```python
from build123d import *

# Parameters (mm, degrees)
F1_DEPTH = 25
F3_DEPTH = 30
F4_W     = 5
F4_H     = 10
F5_DEPTH = 15.001


with BuildPart() as f1:
    # F0 (on Front) → F1 (new body)
    with BuildSketch(Plane.XZ):
        Polygon((0, 80), (0, 0), (15, 0), (15, 35), (75, 35), (75, 80), align=None)
    extrude(amount=-F1_DEPTH)

    # F2 (on face) → F3 (cut)
    with BuildSketch(Plane.XY.offset(80)):
        with BuildLine():
            ThreePointArc((50, 0), (25, 5.456439), (0, 0))
            Line((0, 0), (50, 0))
        make_face()
    extrude(amount=-F3_DEPTH, mode=Mode.SUBTRACT)

    # F4 (on face) → F5 (cut, through all)
    with BuildSketch(Plane.YZ.offset(15)):
        with Locations((22.5, 5)):
            Rectangle(F4_W, F4_H)
    extrude(amount=-F5_DEPTH, mode=Mode.SUBTRACT)


solid = f1.part
```
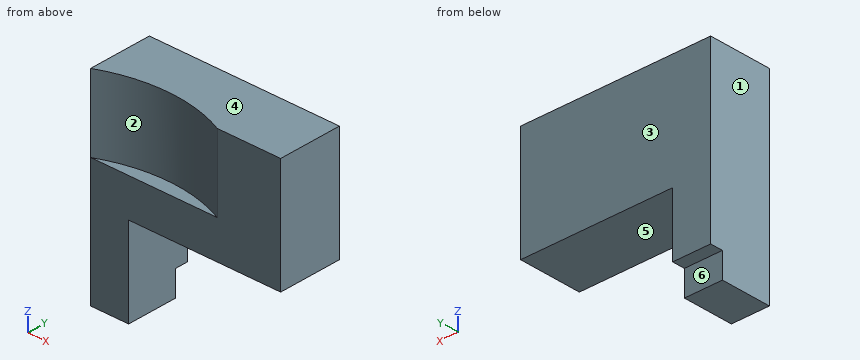
Source: CAD feature listing. Evaluate the final solid. Frame: model axes, mm. Face numbers are marked on the shaded views. A direction names the side the tool comes from. Give positions to 0.01 mm unless a question says otherwise; leave off trailing zeros. Write each loop counter-clockwise with the first axis right and the second up, starting at its lowest first coordinate (ties: lowest second). Pieces come first, ordered by that corner, then holes. Notation, with made-up numbers: (41, 25.25) - (45, 25.25) arc R30 cw to (45, 60.25) - close; hole circle Ø8 at (43, 28). An arc over 180 degrees is marked (long way). One line per item, written item: value. Start each with the question number.
Q1. Section query A-A, the plane y = 21.25. Return the cut outline in (x, z).
Q2. Section query B-B, the plane z = 66.5. Return the cut outline in (x, y).
Q3. Material intervals for probe 1 along Z at (x, y) = (49.5, 18); probe 2 along X at (y, z) = (11.25, 14), sorted ascending. Write a range as from..to.
Q4. Draft query along X for the marked faces 1, 2 and 3. Return one class per face: +X half, -X half, draft (parallel to the pull), parting line (faces both ways), or undercut.
Q5. Section query D-D, the plane z = 22.5. Return the cut outline in (x, y), then the cut area to 3 significant figures.
Q6. Section query C-C, the plane x = 56.5. Return the cut outline in (y, z).
Q7. First-contact query: pin 1 Ø8 at (x, z) = (42, 55) entering from -Y; pin 2 Ø1.6 at (x, y) = (27, 1.5) entering from +Z; pin 3 Ø3 at (x, y) = (65.5, 8.5) entering from -Z. Flat tips, straight axial feed; report the tip coordinate or a pass-through.
Q8. Set-up query: the marked faces 4, 5 and 6. Return all of +Z, -Z, +X, -X, +Y, -Y with unobstructed straight access to the full face (end or side cutting, diameter ignored); none if empty.
Answer:
1. outline: (0, 10) - (15, 10) - (15, 35) - (75, 35) - (75, 80) - (0, 80) - close
2. outline: (0, 0) arc R60 cw to (50, 0) - (75, 0) - (75, 25) - (0, 25) - close
3. probe 1: z = 35..80
3. probe 2: x = 0..15
4. face 1: -X half
4. face 2: undercut
4. face 3: draft
5. outline: (0, 0) - (15, 0) - (15, 25) - (0, 25) - close
5. area: 375 mm2
6. outline: (0, 35) - (25, 35) - (25, 80) - (0, 80) - close
7. pin 1: stops at y = 1.66
7. pin 2: stops at z = 50
7. pin 3: stops at z = 35
8. face 4: +Z, +X, -X, +Y, -Y
8. face 5: -Z, +X, +Y, -Y
8. face 6: -Z, +X, -X, +Y
